Read the model definition and answer for the solid it produces. Units are mm, in the model's axes. A direction names the side the tool comes from. Give positions to 0.01 mm unless a question says otherwise; leave off trailing zeros. Write each loop counter-clockwise with the first axis right and the second up, starting at its lowest first coordinate (ties: lowest second). Pieces come first, ordered by that corner, then holes. Notation, with made-up numbers: (40.25, 60.5) - (45.25, 60.5) arc R19 ccw to (45.25, 78.5) - close; hole circle Ø3 at (24, -19.75). An arc over 180 degrees is marked (long way). Answer as a JSON object with one key per item and string values. Group by question number.
```python
from build123d import *
from OCP.BRepFilletAPI import BRepFilletAPI_MakeChamfer

# Parameters (mm, degrees)
SKETCH1_W           = 13.29305136
SKETCH1_H           = 12
BOSS_EXTRUDE1_DEPTH = 120
SKETCH2_W           = 8.2
SKETCH2_H           = 54.027992046
CUT_EXTRUDE1_DEPTH  = 2
SKETCH3_R           = 1.5
CUT_EXTRUDE2_DEPTH  = 140
SKETCH4_OUTSIDE_W   = 39.56
SKETCH4_OUTSIDE_H   = 38.266
CUT_EXTRUDE3_DEPTH  = 115
CHAMFER1_SIZE       = 1
CHAMFER1_SIZE2      = 5.67128182
CHAMFER2_SIZE       = 2
CHAMFER3_SIZE       = 7
CHAMFER3_SIZE2      = 1.234288865
CHAMFER4_SIZE       = 2
CHAMFER4_SIZE2      = 3.464101615


with BuildPart() as part:
    # Sketch1 → Boss-Extrude1 (new body)
    with BuildSketch(Plane(origin=(0, 0, 0), x_dir=(1, 0, 0), z_dir=(0, 1, 0))):
        Rectangle(SKETCH1_W, SKETCH1_H)
    extrude(amount=BOSS_EXTRUDE1_DEPTH)

    # Sketch2 → Cut-Extrude1 (cut)
    with BuildSketch(Plane.XZ):
        Rectangle(SKETCH2_W, SKETCH2_H)
    extrude(amount=-CUT_EXTRUDE1_DEPTH, mode=Mode.SUBTRACT)

    # Sketch3 → Cut-Extrude2 (cut)
    with BuildSketch(Plane(origin=(0, 120, 0), x_dir=(1, 0, 0), z_dir=(0, 1, 0))):
        with Locations(Location((0, 0, 0), (0, 0, 270))):
            Circle(SKETCH3_R)
    extrude(amount=-CUT_EXTRUDE2_DEPTH, mode=Mode.SUBTRACT)

    # Sketch4 outside → Cut-Extrude3 (cut)
    with BuildSketch(Plane(origin=(0, 120, 0), x_dir=(1, 0, 0), z_dir=(0, 1, 0))):
        Rectangle(SKETCH4_OUTSIDE_W, SKETCH4_OUTSIDE_H)
        Polygon((-2.5, -4.330127019), (2.5, -4.330127019), (5, 0), (2.5, 4.330127019), (-2.5, 4.330127019), (-5, 0), align=None, mode=Mode.SUBTRACT)
    extrude(amount=-CUT_EXTRUDE3_DEPTH, mode=Mode.SUBTRACT)

    # Chamfer1
    chamfer1_edges = [part.edges().sort_by_distance(p)[0] for p in [
        (0, 5, 4.330127019),
        (3.75, 5, 2.165063509),
        (3.75, 5, -2.165063509),
        (0, 5, -4.330127019),
        (-3.75, 5, -2.165063509),
        (-3.75, 5, 2.165063509),
    ]]
    chamfer1_side = [part.faces().sort_by_distance(p)[0] for p in [
        (-6.467443237, 5, 0),
    ]]
    chamfer(chamfer1_edges, length=CHAMFER1_SIZE, length2=CHAMFER1_SIZE2, reference=chamfer1_side[0])

    # Chamfer2
    chamfer2_edges = [part.edges().sort_by_distance(p)[0] for p in [
        (6.64652568, 2.5, 6),
        (-6.64652568, 2.5, 6),
        (-6.64652568, 2.5, -6),
        (6.64652568, 2.5, -6),
    ]]
    chamfer(chamfer2_edges, length=CHAMFER2_SIZE)

    # Chamfer3: one chamfer whose edges measure the first distance from different faces: ONE call of the kernel's chamfer builder (chamfer() names one face for all edges)
    chamfer3_edges_1 = [part.edges().sort_by_distance(p)[0] for p in [
        (3.75, 120, 2.165063509),
    ]]
    chamfer3_side_1 = [part.faces().sort_by_distance(p)[0] for p in [
        (3.75, 65.33564091, 2.165063509),
    ]]
    chamfer3_edges_2 = [part.edges().sort_by_distance(p)[0] for p in [
        (0, 120, 4.330127019),
    ]]
    chamfer3_side_2 = [part.faces().sort_by_distance(p)[0] for p in [
        (0, 65.33564091, 4.330127019),
    ]]
    chamfer3_edges_3 = [part.edges().sort_by_distance(p)[0] for p in [
        (-3.75, 120, 2.165063509),
    ]]
    chamfer3_side_3 = [part.faces().sort_by_distance(p)[0] for p in [
        (-3.75, 65.33564091, 2.165063509),
    ]]
    chamfer3_edges_4 = [part.edges().sort_by_distance(p)[0] for p in [
        (-3.75, 120, -2.165063509),
    ]]
    chamfer3_side_4 = [part.faces().sort_by_distance(p)[0] for p in [
        (-3.75, 65.33564091, -2.165063509),
    ]]
    chamfer3_edges_5 = [part.edges().sort_by_distance(p)[0] for p in [
        (0, 120, -4.330127019),
    ]]
    chamfer3_side_5 = [part.faces().sort_by_distance(p)[0] for p in [
        (0, 65.33564091, -4.330127019),
    ]]
    chamfer3_edges_6 = [part.edges().sort_by_distance(p)[0] for p in [
        (3.75, 120, -2.165063509),
    ]]
    chamfer3_side_6 = [part.faces().sort_by_distance(p)[0] for p in [
        (3.75, 65.33564091, -2.165063509),
    ]]
    chamfer3 = BRepFilletAPI_MakeChamfer(part.part.solid().wrapped)
    for e in chamfer3_edges_1:
        chamfer3.Add(CHAMFER3_SIZE, CHAMFER3_SIZE2, e.wrapped, chamfer3_side_1[0].wrapped)  # the first distance lies on this face
    for e in chamfer3_edges_2:
        chamfer3.Add(CHAMFER3_SIZE, CHAMFER3_SIZE2, e.wrapped, chamfer3_side_2[0].wrapped)  # the first distance lies on this face
    for e in chamfer3_edges_3:
        chamfer3.Add(CHAMFER3_SIZE, CHAMFER3_SIZE2, e.wrapped, chamfer3_side_3[0].wrapped)  # the first distance lies on this face
    for e in chamfer3_edges_4:
        chamfer3.Add(CHAMFER3_SIZE, CHAMFER3_SIZE2, e.wrapped, chamfer3_side_4[0].wrapped)  # the first distance lies on this face
    for e in chamfer3_edges_5:
        chamfer3.Add(CHAMFER3_SIZE, CHAMFER3_SIZE2, e.wrapped, chamfer3_side_5[0].wrapped)  # the first distance lies on this face
    for e in chamfer3_edges_6:
        chamfer3.Add(CHAMFER3_SIZE, CHAMFER3_SIZE2, e.wrapped, chamfer3_side_6[0].wrapped)  # the first distance lies on this face
    add(Compound.cast(chamfer3.Shape()), mode=Mode.REPLACE)

    # Chamfer4: one chamfer whose edges measure the first distance from different faces: ONE call of the kernel's chamfer builder (chamfer() names one face for all edges)
    chamfer4_edges_1 = [part.edges().sort_by_distance(p)[0] for p in [
        (-6.64652568, 0, 0),
    ]]
    chamfer4_side_1 = [part.faces().sort_by_distance(p)[0] for p in [
        (-5.281902175, 0, 0),
    ]]
    chamfer4_edges_2 = [part.edges().sort_by_distance(p)[0] for p in [
        (6.64652568, 0, 0),
    ]]
    chamfer4_side_2 = [part.faces().sort_by_distance(p)[0] for p in [
        (5.281902175, 0, 0),
    ]]
    chamfer4 = BRepFilletAPI_MakeChamfer(part.part.solid().wrapped)
    for e in chamfer4_edges_1:
        chamfer4.Add(CHAMFER4_SIZE, CHAMFER4_SIZE2, e.wrapped, chamfer4_side_1[0].wrapped)  # the first distance lies on this face
    for e in chamfer4_edges_2:
        chamfer4.Add(CHAMFER4_SIZE, CHAMFER4_SIZE2, e.wrapped, chamfer4_side_2[0].wrapped)  # the first distance lies on this face
    add(Compound.cast(chamfer4.Shape()), mode=Mode.REPLACE)


solid = part.part
```
1) Find section B-B, the plane y = 34. Write down the section's boundary in (x, z).
2) Flat-ended cylindrical pins translate along their axes: pin 1 Ø4 at (x, y) = (-2, 41) entering from -Z; pin 2 Ø1.5 at (x, y) = (-1, 49) entering from +Z; pin 3 Ø1 at (y, z) = (0.5, 2.5) entering from -X. Find the tip coordinate at first contact, or state that the pin passes through.
3) Find the intervals of material crossed by line 1 (X direction, y = 95, z = 0); line 2 (Y direction, x = -1.5, z = -3); line 3 (Y direction, x = 3.75, z = 5.25), in increasing order. Write a range as [from, to].
4) For a pull along Z with two mould halves and no side action, classify faces 1 (the flat face through (-3.226, 116.549, 1.822)), 2 (the flat face through (-4.155, 7.875, -2.449)), 3 (the cylindrical face through (0.45, 61.83, 1.43)) as released by +Z, released by -Z, zero draft, split by the parting line, or undercut.
5) Which of the six approach directions +Z, -Z, +X, -X, +Y, -Y give full straight-line access (tool end or side, diameter ignored) to faces 4 (the flat face through (-3.73, 62.55, -2.2)), 5 (the flat face through (0, 63, 4.33)), 6 (the flat face through (-3.77, 62.55, 2.13)), 7 (the flat face through (3.77, 62.55, -2.13)), 8 (the flat face through (0, 63, -4.33))?
6) Find section A-A, the plane x = 0. Write down the section's boundary in (y, z), and give its area (3 significant figures).
Values follow:
{
 "1": {"outline": "(-5, 0) - (-2.5, -4.33) - (2.5, -4.33) - (5, 0) - (2.5, 4.33) - (-2.5, 4.33) - close; hole circle Ø3 at (0, 0)"},
 "2": {"pin 1": "stops at z = -4.33", "pin 2": "stops at z = 4.33", "pin 3": "stops at x = -5.22"},
 "3": {"line 1": "x = [-5, -1.5], [1.5, 5]", "line 2": "y = [2, 120]", "line 3": "y = [2, 5]"},
 "4": {"face 1": "released by +Z", "face 2": "released by -Z", "face 3": "undercut"},
 "5": {"face 4": "-Z, -X, +Y", "face 5": "+Z, +X, -X, +Y", "face 6": "+Z, -X, +Y", "face 7": "-Z, +X, +Y", "face 8": "-Z, +X, -X, +Y"},
 "6": {"outline": "(2, -6) - (5, -6) - (5, -5.33) - (10.67, -4.33) - (113, -4.33) - (120, -3.1) - (120, -1.5) - (2, -1.5) - close; (2, 1.5) - (120, 1.5) - (120, 3.1) - (113, 4.33) - (10.67, 4.33) - (5, 5.33) - (5, 6) - (2, 6) - close", "area": "675 mm2"}
}
